from build123d import *

# Parameters (mm, degrees)
F1_DEPTH = 15
F2_DEPTH = 10
F3_DEPTH = 10
F4_W     = 15
F4_H     = 10
F5_DEPTH = 0.01
F6_W     = 15
F6_H     = 4
F7_DEPTH = 0.01
F8_W     = 12
F8_H     = 12


with BuildPart() as f1:
    # F0 (on Front) → F1 (new body)
    with BuildSketch(Plane.XZ):
        with BuildLine():
            Line((-105, 0), (-120, 0))
            ThreePointArc((-120, 0), (-84.8528137424, -84.8528137424), (0, -120))
            Line((0, -120), (0, -105))
            ThreePointArc((0, -105), (-74.2462120246, -74.2462120246), (-105, 0))
        make_face()
    extrude(amount=F1_DEPTH)

    # F2 (add): a face of the model
    f2_faces = [f1.faces().sort_by_distance(p)[0] for p in [
        (-112.5, -7.5, 0),
    ]]
    extrude(f2_faces, amount=F2_DEPTH)

    # F3 (add): a face of the model
    f3_faces = [f1.faces().sort_by_distance(p)[0] for p in [
        (0, -7.5, -112.5),
    ]]
    extrude(f3_faces, amount=F3_DEPTH)

    # F4 (on face) → F5 (join)
    with BuildSketch(Plane.XZ.offset(15)):
        with Locations((-112.5, 5)):
            Rectangle(F4_W, F4_H)
    extrude(amount=F5_DEPTH)

    # F6 (on face) → F7 (cut)
    with BuildSketch(Plane.XZ.offset(15.01)):
        with Locations((-112.5, 8)):
            Rectangle(F6_W, F6_H)
    extrude(amount=-F7_DEPTH, mode=Mode.SUBTRACT)

    # F9: sweep along a path in F9_path
    with BuildLine(Plane(origin=(-105, 0, 0), x_dir=(0, 0, -1), z_dir=(0, 1, 0))) as f9_path:
        Line((-10, 0), (0, 0))
        ThreePointArc((0, 0), (74.2462120246, -30.7537879754), (105, -105))
        Line((105, -105), (105, -115))
    # F8 (on face) → F9 (sweep, cut)
    with BuildSketch(Plane.YZ.offset(10)):
        with Locations((-7.5, -112.5)):
            Rectangle(F8_W, F8_H)
    sweep(path=f9_path.line, mode=Mode.SUBTRACT)


solid = f1.part
Design review of the part built by this model. Coordinates are the model's own, in mm. A direction names the side the tool comes from. Round coordinates to 2 decimals unless told otherwise and drop trailing zeros. Loops run counter-clockwise (first coordinate to the right, second up) from the corner with the lowest first, then second, coordinate; pieces in that order, holes last. Notation, with made-up numbers: (4.5, 78.25) -> (54.5, 78.25) arc R22 ccw to (54.5, 110.25) -> close; hole circle Ø3 at (1.5, 63). An arc over 180 degrees is marked (long way). Use one line per item in the form item = value. Start each with the question number.
Q1. Machinability: for faces 5 (the face through (-73, -13.5, -78)), 6 (the face through (5, -7, -106.5)), 7 (the face through (-106.5, -7, 5)), which of the approach directions +Z, -Z, +X, -X, +Y, -Y give a long, thin tool a straight path to every point of the face, cutting with its end or side? Answer none if there is none.
Q2. We need section B-B on z = -93. Give the boundary of the cut face in (x, y), then the cut area to 3 significant figures.
Q3. We need section A-A on y = -3.75. Give the boundary of the cut face in (x, z).
Q4. Wall thickness on line 1 along Z through (x, y) = (-1, -5.75); line 2 along Y through (x, z) = (-83, -72); line 3 along Z through (x, y) = (-77.5, -7): over which ranges is each line inside the solid? List them lowest first. Write a range as [from, to].
Q5. We need section C-C on x = -87. Give the boundary of the cut face in (y, z), then the cut area to 3 significant figures.
Q6. Draft analysis for pull direction Y (two halves, no side actions). For faces 1 (the face through (-75, -15, -78)), 2 (the face through (5, -8, -118.5)), 3 (the face through (-74, -1.5, -78)), 4 (the face through (-120, -7, 5)), state which applies: +Y half, -Y half, draft (parallel to the pull), parting line (faces both ways), or undercut.
Q7. For pin 1 Ø5 at (y, z) = (-10, -75) entering from -X; pin 2 Ø3 at (y, z) = (-7.5, 4) entering from +X; pin 3 Ø3 at (x, y) = (-55, -5.5) entering from -Z, all flat-tipped, find the tip position at first contact; note any pin that passes through.
Calculated:
q1.face_5 = none
q1.face_6 = +X
q1.face_7 = +Z
q2.outline = (-75.84, -15) -> (-48.74, -15) -> (-48.74, 0) -> (-75.84, 0) -> close; hole (-73.44, -13.5) -> (-51.9, -13.5) -> (-51.9, -1.5) -> (-73.44, -1.5) -> close
q2.area = 148 mm²
q3.outline = (-120, 0) arc R120 ccw to (0, -120) -> (10, -120) -> (10, -118.5) -> (0, -118.5) arc R118.5 cw to (-118.5, 0) -> (-118.5, 10) -> (-120, 10) -> close; (-106.5, 0) arc R106.5 ccw to (0, -106.5) -> (10, -106.5) -> (10, -105) -> (0, -105) arc R105 cw to (-105, 0) -> (-105, 10) -> (-106.5, 10) -> close
q4.line_1 = [-120, -118.5], [-106.5, -105]
q4.line_2 = [-15, -13.5], [-1.5, 0]
q4.line_3 = [-91.62, -89.64], [-73.05, -70.84]
q5.outline = (-15, -82.65) -> (0, -82.65) -> (0, -58.79) -> (-15, -58.79) -> close; hole (-13.5, -80.46) -> (-1.5, -80.46) -> (-1.5, -61.43) -> (-13.5, -61.43) -> close
q5.area = 130 mm²
q6.face_1 = -Y half
q6.face_2 = undercut
q6.face_3 = undercut
q6.face_4 = draft
q7.pin_1 = -95.62
q7.pin_2 = -105
q7.pin_3 = -107.41
